```python
from build123d import *

# Parameters (mm, degrees)
F1_R      = 4
F1_R_2    = 8.5
F2_DEPTH  = 2
F4_DEPTH  = 6
F5_R      = 0.8
F6_DEPTH  = 4.618034
F8_DEPTH  = 8
F9_R      = 1.4
F10_DEPTH = 10
F11_R     = 2
F12_DEPTH = 3
F13_W     = 9.5
F13_H     = 9.5
F13_R     = 4
F14_DEPTH = 1
F15_R     = 0.9
F16_DEPTH = 5


with BuildPart() as f2:
    # F1 (on Front) → F2 (new body)
    with BuildSketch(Plane.XZ):
        Polygon((-22, 25.5), (-22, 0.118034), (-19.690983, -4.5), (19.690983, -4.5), (22, 0.118034), (22, 25.5), align=None)
        with Locations((-12.3, 13)):
            Circle(F1_R, mode=Mode.SUBTRACT)
        with Locations((10.94, 11.55)):
            Circle(F1_R_2, mode=Mode.SUBTRACT)
    extrude(amount=F2_DEPTH)

    # F3 (on face) → F4 (join)
    with BuildSketch(Plane(origin=(0, 0, 0), x_dir=(-1, 0, 0), z_dir=(0, 1, 0))):
        Polygon((22, 0.118034), (-22, 0.118034), (-19.690983, -4.5), (19.690983, -4.5), align=None)
    extrude(amount=F4_DEPTH)

    # F5 (on face) → F6 (cut, through all)
    with BuildSketch(Plane(origin=(0, 0, -4.5), x_dir=(1, 0, 0), z_dir=(0, 0, -1))):
        with Locations((-17, -1)):
            Circle(F5_R)
        with Locations((17, -1)):
            Circle(F5_R)
    extrude(amount=-F6_DEPTH, mode=Mode.SUBTRACT)

    # F7 (on face) → F8 (join)
    with BuildSketch(Plane(origin=(0, 0, 0), x_dir=(-1, 0, 0), z_dir=(0, 1, 0))):
        with BuildLine():
            ThreePointArc((-17.408219, 17.06472), (-15.997514, 18.381658), (-14.326099, 19.346431))
            ThreePointArc((-14.326099, 19.346431), (-19.025005, 22.471173), (-17.408219, 17.06472))
        make_face()
        with BuildLine():
            ThreePointArc((-4.471781, 6.03528), (-5.882486, 4.718342), (-7.553901, 3.753569))
            ThreePointArc((-7.553901, 3.753569), (-7.618397, 3.399372), (-7.64, 3.04))
            Line((-7.64, 3.04), (-7.64, 0.118034))
            Line((-7.64, 0.118034), (-2.4, 0.118034))
            Line((-2.4, 0.118034), (-2.4, 5.035595))
            ThreePointArc((-2.4, 5.035595), (-3.336266, 5.741903), (-4.471781, 6.03528))
        make_face()
    extrude(amount=F8_DEPTH)

    # F9 (on face) → F10 (cut, through all)
    with BuildSketch(Plane(origin=(0, 8, 0), x_dir=(-1, 0, 0), z_dir=(0, 1, 0))):
        with Locations((-17.24, 20.06)):
            Circle(F9_R)
        with Locations((-4.64, 3.04)):
            Circle(F9_R)
    extrude(amount=-F10_DEPTH, mode=Mode.SUBTRACT)

    # F11 (on face) → F12 (join)
    with BuildSketch(Plane(origin=(0, 0, 0), x_dir=(-1, 0, 0), z_dir=(0, 1, 0))):
        with Locations((-0.1, 23.5)):
            Circle(F11_R)
        with Locations((12.4, 23.5)):
            Circle(F11_R)
        with BuildLine():
            Line((1.9, 0.118034), (1.9, 2.5))
            ThreePointArc((1.9, 2.5), (1.144335, 4.065768), (-0.55163, 4.44834))
            ThreePointArc((-0.55163, 4.44834), (-1.556353, 4.488475), (-2.4, 5.035595))
            Line((-2.4, 5.035595), (-2.4, 0.118034))
            Line((-2.4, 0.118034), (1.9, 0.118034))
        make_face()
        with BuildLine():
            Line((14.4, 0.118034), (14.4, 2.5))
            ThreePointArc((14.4, 2.5), (12.4, 4.5), (10.4, 2.5))
            Line((10.4, 2.5), (10.4, 0.118034))
            Line((10.4, 0.118034), (14.4, 0.118034))
        make_face()
    extrude(amount=F12_DEPTH)

    # F13 (on face) → F14 (cut)
    with BuildSketch(Plane(origin=(0, 0, 0), x_dir=(-1, 0, 0), z_dir=(0, 1, 0))):
        with Locations((12.3, 13)):
            Rectangle(F13_W, F13_H)
        with Locations((12.3, 13)):
            Circle(F13_R, mode=Mode.SUBTRACT)
    extrude(amount=-F14_DEPTH, mode=Mode.SUBTRACT)

    # F15 (on face) → F16 (cut, through all)
    with BuildSketch(Plane(origin=(0, 3, 0), x_dir=(-1, 0, 0), z_dir=(0, 1, 0))):
        with Locations((-0.1, 23.5)):
            Circle(F15_R)
        with Locations((12.4, 23.5)):
            Circle(F15_R)
        with Locations((-0.1, 2.5)):
            Circle(F15_R)
        with Locations((12.4, 2.5)):
            Circle(F15_R)
    extrude(amount=-F16_DEPTH, mode=Mode.SUBTRACT)


solid = f2.part
```
Could you check a few things on this model? Use its own coordinates, in mm. A direction names the side the tool comes from. Round coordinates to 2 decimals unless told otherwise and drop trailing zeros. Loops run counter-clockwise (first coordinate to the right, second up) from the corner with the lowest first, then second, coordinate; pieces in that order, holes last. Notation, with made-up numbers: M 36.25,83.25 L 52.25,83.25 A20 ccw 52.25,97.25 Z; hole C 13.5,-34.75 d6. An arc over 180 degrees is marked long. Write item = value, one per line.
1. I need wall thicknesses on probe 1 along Z at (x, y) = (-12.3, -1.3); probe 2 along Z at (x, y) = (0.1, 1.5); probe 3 along Z at (x, y) = (16.5, 5.25). Which ranges of each line are inside material? Lowest first, please.
Results below:
probe_1 = -4.5 to 1.61, 3.39 to 9, 17 to 22.61, 24.39 to 25.5
probe_2 = -4.5 to 1.6, 3.4 to 4.5, 21.5 to 22.6, 24.4 to 25.5
probe_3 = -4.5 to 0.12, 17.98 to 18.87, 21.25 to 22.97
2. I want a section at C-C, the plane x = 10.94. Write out the boundary of the cut face in (y, z), and give its area (3 significant figures).
Results below:
outline = M -2,-4.5 L 6,-4.5 L 6,0.12 L 0,0.12 L 0,3.05 L -2,3.05 Z; M -2,20.05 L 0,20.05 L 0,25.5 L -2,25.5 Z
area = 53.7 mm²
3. Thinking about a two-plate mould opening in Z: for faces 6 (the face through (3.321, 3.944, 5.735)), 7 (the face through (-12.4, 1.5, 4.5)), 8 (the face through (0.8, 3, 1.5)), which applies, +Z half, -Z half, draft (parallel to the pull), parting line (faces both ways), or undercut?
Results below:
face_6 = +Z half
face_7 = undercut
face_8 = draft
4. I want a section at D-D, the plane y = 2.25. Count the separate pieces of the cut face and the enclosed holes in it, and give its area (3 significant figures).
Results below:
separate_pieces = 4
enclosed_holes = 6
area = 281 mm²
5. Will these pins go through, and if not, where does the flat tip stop? P1, Ø3, axis at x = 0.1, z = 23.5, coming from the +Y side; P2, Ø1.8, axis at x = -17, y = 1, coming from the +Z side; P3, Ø4, axis at y = 4.5, z = 2.5, coming from the -X side.
Results below:
P1 = 3
P2 = 0.12
P3 = -14.4
6. I want a section at A-A, the plane y = 7. Write out the boundary of the cut face in (x, z).
Results below:
outline = M 2.4,0.12 L 7.64,0.12 L 7.64,3.04 A3 ccw 7.55,3.75 A8.5 cw 4.47,6.04 A3 ccw 2.4,5.04 Z; M 14.33,19.35 A8.5 cw 17.41,17.06 A3 ccw long Z; hole C 4.64,3.04 d2.8; hole C 17.24,20.06 d2.8
7. Which directions (+Z, -Z, +X, -X, +Y, -Y) give clear straight access to the entire face, cutting with the end or side of a thin tool? Please do faces 1 (the face through (0, 2, -4.5)), 2 (the face through (-1, 3, 23)), 3 (the face through (-12.2, -1, 17.3)), 4 (the face through (5, 7, 0.118)), 5 (the face through (7.64, 4, 2)).
Results below:
face_1 = -Z, +X, -X, +Y, -Y
face_2 = +Z, -X, +Y
face_3 = +Y
face_4 = -Z, +X, -X, +Y
face_5 = +Z, +X, +Y
8. I want a section at B-B, the plane z = 23.5. Write out the boundary of the cut face in (x, y), and give its area (3 significant figures).
Results below:
outline = M -22,-2 L -13.3,-2 L -13.3,3 L -14.4,3 L -14.4,0 L -22,0 Z; M -11.5,-2 L -0.8,-2 L -0.8,3 L -1.9,3 L -1.9,0 L -10.4,0 L -10.4,3 L -11.5,3 Z; M 1,-2 L 22,-2 L 22,0 L 2.1,0 L 2.1,3 L 1,3 Z
area = 94.0 mm²
